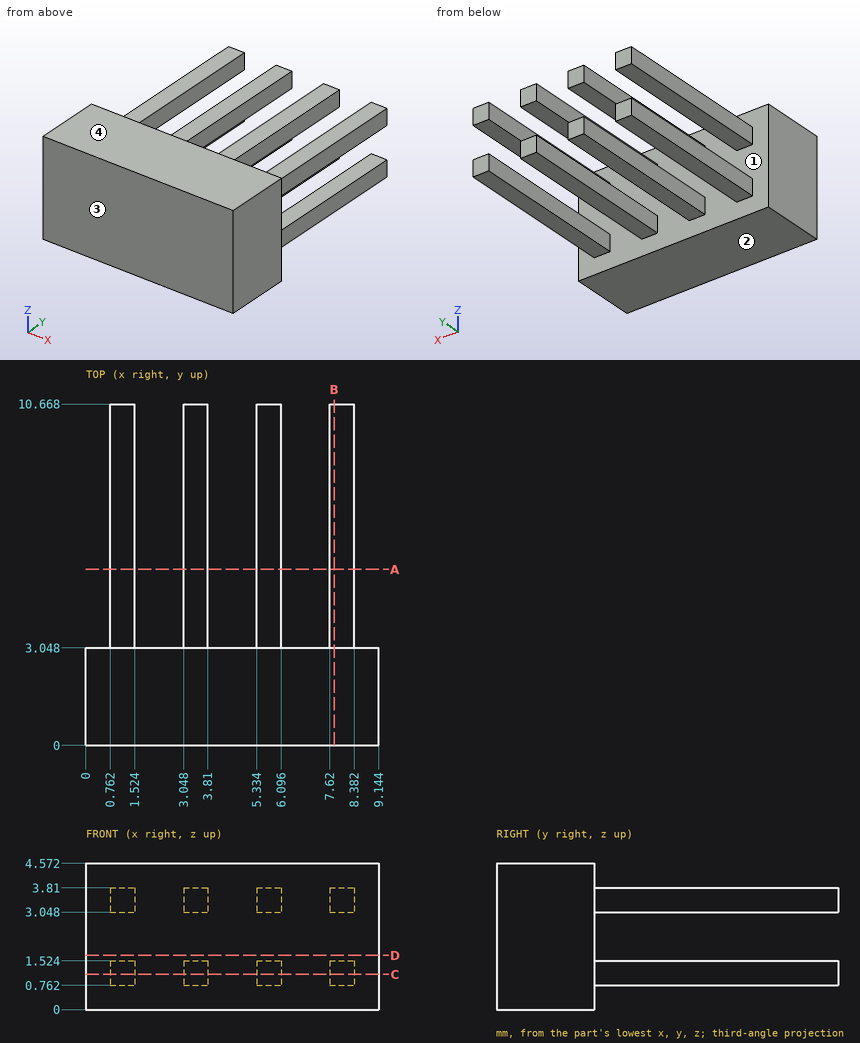
Source: three-view drawing plus pictorial views. Frame: mm from the lowest corner of the part. Coordinates: 2 decimals unless noted, no trailing zeros. Loops run counter-clockwise (first coordinate to the right, second up) from the corner with the lowest first, then second, coordinate; pieces in that order, holes last. Notation, with made-up numbers: (16, 75) - (24, 75) arc R20 cw to (24, 80) - close; hole circle Ø7 at (60, 63). An arc over 180 degrees is marked (long way). Answer in a Markdown table with one row per item. Add a question column.
Item 1: Section query A-A on y = 5.5. State how many separate pieces and enclosed holes the cut face has, then the cut area to 3 significant figures.
Item 2: Line query: line 1 along X through (y, z) = (5.5, 3.4); line 2 along Z through (x, y) = (7.75, 6.25); line 3 along Y through (x, z) = (8.75, 2.8). Output: solid intervals per line, ascending. Write a range as [from, to].
Item 3: Section query C-C on z = 1.1. Return the cut outline in (x, y).
Item 4: Mould query, pull axis Z, two halves, no side actions, for the marked faces 1, 2, 3 and 4. Classes: released by +Z, released by -Z, zero draft, split by the parting line, or undercut.
Item 5: Section query D-D on z = 1.7. Return the cut outline in (x, y).
Item 6: Section query B-B on x = 7.75. Return the cut outline in (y, z), then the cut area to 3 significant figures.
Item 7: Contact query for flat-ended pins moving along their axis: P1, Ø0.6, axis at y = 8.5, z = 1, coming from the +X side; P2, Ø0.6, axis at x = 1.5, y = 9, coming from the -Z side; P3, Ø1, axis at y = 7.5, z = 2.5, coming from the +X side; P4, Ø0.6, axis at x = 8, y = 6, coming from the +Z side. Output: stop coordinate, or through.
Recorded:
| question | item | result |
|---|---|---|
| 1 | separate pieces | 8 |
| 1 | enclosed holes | 0 |
| 1 | area | 4.65 mm^2 |
| 2 | line 1 | [0.76, 1.52], [3.05, 3.81], [5.33, 6.1], [7.62, 8.38] |
| 2 | line 2 | [0.76, 1.52], [3.05, 3.81] |
| 2 | line 3 | [0, 3.05] |
| 3 | outline | (0, 0) - (9.14, 0) - (9.14, 3.05) - (8.38, 3.05) - (8.38, 10.67) - (7.62, 10.67) - (7.62, 3.05) - (6.1, 3.05) - (6.1, 10.67) - (5.33, 10.67) - (5.33, 3.05) - (3.81, 3.05) - (3.81, 10.67) - (3.05, 10.67) - (3.05, 3.05) - (1.52, 3.05) - (1.52, 10.67) - (0.76, 10.67) - (0.76, 3.05) - (0, 3.05) - close |
| 4 | face 1 | undercut |
| 4 | face 2 | released by -Z |
| 4 | face 3 | zero draft |
| 4 | face 4 | released by +Z |
| 5 | outline | (0, 0) - (9.14, 0) - (9.14, 3.05) - (0, 3.05) - close |
| 6 | outline | (0, 0) - (3.05, 0) - (3.05, 0.76) - (10.67, 0.76) - (10.67, 1.52) - (3.05, 1.52) - (3.05, 3.05) - (10.67, 3.05) - (10.67, 3.81) - (3.05, 3.81) - (3.05, 4.57) - (0, 4.57) - close |
| 6 | area | 25.5 mm^2 |
| 7 | P1 | x = 8.38 |
| 7 | P2 | z = 0.76 |
| 7 | P3 | through |
| 7 | P4 | z = 3.81 |
